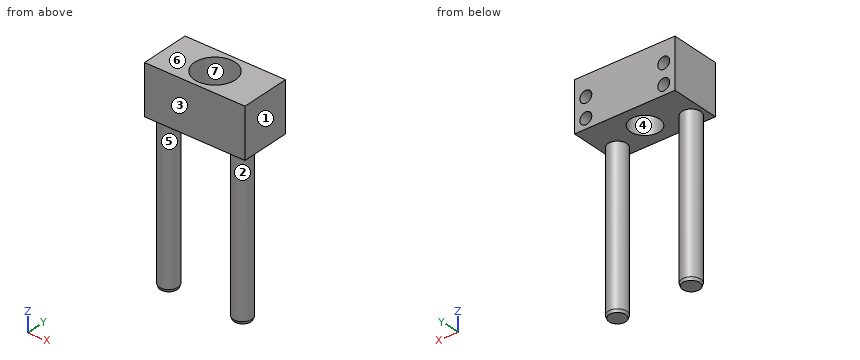
Autodesk Inventor part; units mm, degrees
ref_plane "YZ Plane" through (0, 0, 0) normal (1, 0, 0) x (0, 1, 0)
ref_plane "XZ Plane" through (0, 0, 0) normal (0, 1, 0) x (-1, 0, 0)
ref_plane "XY Plane" through (0, 0, 0) normal (0, 0, 1) x (1, 0, 0)
sketch "Sketch1" plane through (0, 0, 0) normal (0, 1, 0) x (-1, 0, 0)
  line L0 (12.71, 0) -> (12.71, 12.6)
  line L1 (12.71, 12.6) -> (-12.71, 12.6)
  line L2 (-12.71, 12.6) -> (-12.71, 0)
  line L3 (-12.71, 0) -> (12.71, 0)
  point P0 (0, 0)
  dimension "d0" = 12.71
  dimension "d1" = 12.6
  dimension "d2" = 25.42
extrude "Extrusion1" add sketch "Sketch1" along normal mid plane 12.56
sketch "Sketch2" plane through (-12.71, 6.28, 12.6) normal (0, 0, 1) x (1, 0, 0)
  circle A0 centre (12.71, -6.28) radius 3.7
  dimension "d5" = 7.4
extrude "Extrusion2" cut sketch "Sketch2" against normal blind 17.3225
sketch "Sketch3" plane through (-12.71, 6.28, 12.6) normal (0, 0, 1) x (1, 0, 0)
  circle A0 centre (12.71, -6.28) radius 5.15
  dimension "d8" = 10.3
extrude "Extrusion3" cut sketch "Sketch3" against normal blind 6.5
sketch "Sketch4" plane through (0, 6.28, 0) normal (0, 1, 0) x (1, 0, 0)
  line L0 (0, 0) -> (-9.85, 0) construction
  line L1 (-9.85, 0) -> (-9.85, -2.5) construction
  circle A0 centre (-9.85, -2.5) radius 1.5
  line L2 (-9.85, -2.5) -> (-9.85, -7.5) construction
  circle A1 centre (-9.85, -7.5) radius 1.5
  circle A2 centre (9.85, -2.5) radius 1.5
  circle A3 centre (9.85, -7.5) radius 1.5
  dimension "d11" = 9.85
  dimension "d12" = 2.5
  dimension "d13" = 3
  dimension "d14" = 5
  dimension "d15" = 3
extrude "Extrusion4" cut sketch "Sketch4" against normal blind 8.2
chamfer "Chamfer1" distance 0.25 angle 45 4 edges at (-11.35, -1.92, 7.5) (-11.35, -1.92, 2.5) (8.35, -1.92, 2.5) (8.35, -1.92, 7.5)
sketch "Sketch5" plane through (12.71, 6.28, 0) normal (0, 0, -1) x (-1, 0, 0)
  line L0 (1, -12.56) -> (1, -9.185) construction
  line L1 (1, -9.185) -> (3.375, -9.185) construction
  circle A0 centre (3.375, -9.185) radius 2.375
  circle A1 centre (12.71, -6.28) radius 3.7
  line L2 (12.71, -12.56) -> (12.71, -6.28) construction
  circle A2 centre (22.045, -9.185) radius 2.375
  point P0 (0, -12.56)
  dimension "d21" = 1
  dimension "d22" = 3.375
  dimension "d23" = 2.375
extrude "Extrusion5" add sketch "Sketch5" along normal blind 39.6 contours A0 | A2
chamfer "Chamfer2" distance 0.25 angle 70 1 edges at (11.71, -2.905, -39.6) measured on face at (9.5733, -3.5643, -39.6)
chamfer "Chamfer3" distance 0.25 angle 70 1 edges at (-6.96, -2.905, -39.6) measured on face at (-9.9756, -2.2535, -39.6)
properties part number "PocketNC_Vise_part1" material "Aluminum 6061"
Input: part model. Units: mm. Frame: model coordinates. Face numbers are marked on the shaded views. A direction names the side the tool comes from. Give positions to 0.01 mm unless a question says otherwise; leave off trailing zeros. Write each loop counter-clockwise with the first axis right and the second up, starting at its lowest first coordinate (ties: lowest second). Pieces come first, ordered by that corner, then holes. Notation, with made-up numbers: (25, -33.5) -> (79, -33.5) arc R22 cw to (79, -6.5) -> close; hole circle Ø5 at (14, 4). An arc over 180 degrees is marked (long way). Use one line per item in the form item = value. Start each with the question number.
1) Draft query along Y for the marked faces 1, 2, 3 and 4. Return one class per face: pulls with the +Y half, pulls with the -Y half, needs draft (parallel to the pull), parting line crosses it, or undercut.
2) Section query B-B on x = 0. Return the cut outline in (y, z), then the cut area to 3 significant figures.
3) Section query D-D on y = 2.25. Return the cut outline in (x, z).
4) Section query A-A on y = 0. Return the cut outline in (x, z).
5) Set-up query: the marked faces 5, 6 and 7. Return all of +Z, -Z, +X, -X, +Y, -Y with unobstructed straight access to the full face (end or side cutting, diameter ignored); none if empty.
6) Ray query, probe 1 along Z at (x, y) = (9.85, 4.25); probe 2 along Y at (x, z) = (0, 2); probe 3 along X at (y, z) = (-3, -31). Return the intervals inside material, ascending. Write a range as from..to.
7) Pin query (flat end, axial travel): pin 1 (4 mm diameter, centred on x = -9.85, z = 7.5, fed in from +Y); pin 2 (6 mm diameter, centred on y = -1.5, z = -9.5, fed in from -X); pin 3 (0.8 mm diameter, centred on x = 9.5, z = 7.5, fed in from +Y); pin 4 (8 mm diameter, centred on x = -7, z = -9.5, fed in from +Y). Return the tip coordinate at first contact, or that it passes through.
8) Section query C-C on z = 2.5. Return the cut outline in (x, y), then the cut area to 3 significant figures.
Outcome:
q1.face_1 = needs draft
q1.face_2 = parting line crosses it
q1.face_3 = pulls with the -Y half
q1.face_4 = undercut
q2.outline = (-6.28, 0) -> (-3.7, 0) -> (-3.7, 6.1) -> (-5.15, 6.1) -> (-5.15, 12.6) -> (-6.28, 12.6) -> close; (3.7, 0) -> (6.28, 0) -> (6.28, 12.6) -> (5.15, 12.6) -> (5.15, 6.1) -> (3.7, 6.1) -> close
q2.area = 46.2 mm^2
q3.outline = (-12.71, 0) -> (-2.94, 0) -> (-2.94, 6.1) -> (-4.63, 6.1) -> (-4.63, 12.6) -> (-12.71, 12.6) -> close; (2.94, 0) -> (12.71, 0) -> (12.71, 12.6) -> (4.63, 12.6) -> (4.63, 6.1) -> (2.94, 6.1) -> close; hole circle Ø3 at (-9.85, 2.5); hole circle Ø3 at (-9.85, 7.5); hole circle Ø3 at (9.85, 2.5); hole circle Ø3 at (9.85, 7.5)
q4.outline = (-12.71, 0) -> (-3.7, 0) -> (-3.7, 6.1) -> (-5.15, 6.1) -> (-5.15, 12.6) -> (-12.71, 12.6) -> close; (3.7, 0) -> (12.71, 0) -> (12.71, 12.6) -> (5.15, 12.6) -> (5.15, 6.1) -> (3.7, 6.1) -> close; hole circle Ø3 at (-9.85, 2.5); hole circle Ø3 at (-9.85, 7.5); hole circle Ø3 at (9.85, 2.5); hole circle Ø3 at (9.85, 7.5)
q5.face_5 = -Z
q5.face_6 = +Z, +X, -X, +Y, -Y
q5.face_7 = +Z
q6.probe_1 = 0..1, 4..6, 9..12.6
q6.probe_2 = -6.28..-3.7, 3.7..6.28
q6.probe_3 = -11.71..-6.96, 6.96..11.71
q7.pin_1 = 6.28
q7.pin_2 = -11.71
q7.pin_3 = -1.92
q7.pin_4 = -0.53
q8.outline = (-12.71, -6.28) -> (12.71, -6.28) -> (12.71, 6.28) -> (11.35, 6.28) -> (11.35, -1.67) -> (11.1, -1.92) -> (8.6, -1.92) -> (8.35, -1.67) -> (8.35, 6.28) -> (-8.35, 6.28) -> (-8.35, -1.67) -> (-8.6, -1.92) -> (-11.1, -1.92) -> (-11.35, -1.67) -> (-11.35, 6.28) -> (-12.71, 6.28) -> close; hole circle Ø7.4 at (0, 0)
q8.area = 227 mm^2
